Build history of the part. All positions in model axes, mm. A direction names the side the tool comes from. Round coordinates to 2 decimals unless told otherwise and drop trailing zeros. Write each loop counter-clockwise with the first axis right and the second up, starting at its lowest first coordinate (ties: lowest second). Pieces come first, ordered by that corner, then holes. Notation, with made-up numbers: (15, 24.5) -> (57, 24.5) arc R22 cw to (57, 39.5) -> close; hole circle Ø4 at (66, 70.5). An arc over 180 degrees is marked (long way). Answer as CSV lines item,"result".
from build123d import *

# Parameters (mm, degrees)
BOSS_EXTRUDE1_DEPTH = 6.35
FILLET1_R           = 5


with BuildPart() as part:
    # Sketch1 → Boss-Extrude1 (new body)
    with BuildSketch(Plane(origin=(0, 0, 0), x_dir=(1, 0, 0), z_dir=(0, 1, 0))):
        Polygon((-57.825, 26.738412941), (-42.825, 26.738412941), (-9.574489714, 0), (-42.825, -26.738412941), (-57.825, -26.738412941), (-57.825, -46.5), (-33.250510286, -46.5), (-33.250510286, -34.437743191), (0, -7.69933025), (33.250510286, -34.437743191), (33.250510286, -46.5), (57.825, -46.5), (57.825, -26.738412941), (42.825, -26.738412941), (9.574489714, 0), (42.825, 26.738412941), (57.825, 26.738412941), (57.825, 46.5), (33.250510286, 46.5), (33.250510286, 34.437743191), (0, 7.69933025), (-33.250510286, 34.437743191), (-33.250510286, 46.5), (-57.825, 46.5), align=None)
    extrude(amount=BOSS_EXTRUDE1_DEPTH)

    # Fillet1
    fillet1_edges = [part.edges().sort_by_distance(p)[0] for p in [
        (-33.250510286, 3.175, -34.437743191),
        (0, 3.175, -7.69933025),
        (33.250510286, 3.175, -34.437743191),
        (42.825, 3.175, -26.738412941),
        (9.574489714, 3.175, 0),
        (42.825, 3.175, 26.738412941),
        (33.250510286, 3.175, 34.437743191),
        (0, 3.175, 7.69933025),
        (-33.250510286, 3.175, 34.437743191),
        (-42.825, 3.175, 26.738412941),
        (-9.574489714, 3.175, 0),
    ]]
    fillet(fillet1_edges, radius=FILLET1_R)


solid = part.part
1. Mould opens along X. For faces 5 (the cylindrical face through (-32.746, 3.219, -34.645)), 6 (the cylindrical face through (-12.554, 3.219, -0.063)), 7 (the flat face through (-50, 3, -26.738)) say: +X half, -X half, draft (parallel to the pull), parting line (faces both ways), or undercut.
Results found:
face 5,"undercut"
face 6,"-X half"
face 7,"draft"
2. Cut at C-C, the plane x = -5. Write the cut outline in (y, z).
Results found:
outline,"(0, -11.72) -> (6.35, -11.72) -> (6.35, 11.72) -> (0, 11.72) -> close"
3. Cut at D-D, the plane z = 0.5. Write the cut outline in (x, y), then the cut area to 3 significant figures.
Results found:
outline,"(-12.58, 0) -> (12.58, 0) -> (12.58, 6.35) -> (-12.58, 6.35) -> close"
area,"160 mm2"
4. Drop a flat-ended pin along its axis: pin 1 Ø3 at (x, y) = (23, 5.5) entering from +Z. Give the stop position or say it passes through.
Results found:
pin 1,"stops at z = 27.4"
5. Cut at A-A, the plane z = 40. Write the cut outline in (x, y) (3 decimals).
Results found:
outline,"(-57.825, 0) -> (-33.251, 0) -> (-33.251, 6.35) -> (-57.825, 6.35) -> close; (33.251, 0) -> (57.825, 0) -> (57.825, 6.35) -> (33.251, 6.35) -> close"
6. Which spindle directions (+Z, -Z, +X, -X, +Y, -Y) get a long thin tool onto all of the face, cutting with end or side? Do faces 1 (the flat face through (-33.251, 3, -42)), 2 (the cylindrical face through (-32.773, 3.219, 34.701)), 3 (the flat face through (45, 3, 46.5)), 4 (the flat face through (51, 3, -26.738)). Say none if no direction does.
Results found:
face 1,"-Z, +Y, -Y"
face 2,"+Z, +Y, -Y"
face 3,"+Z, +X, -X, +Y, -Y"
face 4,"+X, +Y, -Y"
7. Cut at B-B, the plane x = -38. Write the cut outline in (y, z).
Results found:
outline,"(0, -46.5) -> (6.35, -46.5) -> (6.35, -22.86) -> (0, -22.86) -> close; (0, 22.86) -> (6.35, 22.86) -> (6.35, 46.5) -> (0, 46.5) -> close"
8. Probe line 1 along X through (y, z) = (4.25, -28.5) (3 decimals); line 2 along Z through (x, y) = (-25, 5.25); line 3 along X through (y, z) = (2.75, 17.5). List the from-to ranges inside material, lowest first.
Results found:
line 1,"x = -57.825 to -25.867, 25.867 to 57.825"
line 2,"z = -27.8 to -12.4, 12.4 to 27.8"
line 3,"x = -31.34 to -12.19, 12.19 to 31.34"
